from build123d import *

# Parameters (mm, degrees)
F0_W     = 41.1972631226
F0_H     = 41.1972631226
F1_DEPTH = 5
F0_R     = 1.65
F2_DEPTH = 2
F4_DEPTH = 4
F5_R     = 14.2181252649
F6_DEPTH = 1.001
F7_R     = 5


with BuildPart() as f1:
    # F0 (on Top) → F1 (new body)
    with BuildSketch(Plane.XY):
        Rectangle(F0_W, F0_H)
        Polygon((-16.9243157806, -12.35), (-13.5756842194, -12.35), (-11.9013684387, -15.25), (-13.5756842194, -18.15), (-16.9243157806, -18.15), (-18.5986315613, -15.25), align=None, mode=Mode.SUBTRACT)
        Polygon((13.5756842194, -12.35), (16.9243157806, -12.35), (18.5986315613, -15.25), (16.9243157806, -18.15), (13.5756842194, -18.15), (11.9013684387, -15.25), align=None, mode=Mode.SUBTRACT)
        Polygon((-18.5986315613, 15.25), (-16.9243157806, 18.15), (-13.5756842194, 18.15), (-11.9013684387, 15.25), (-13.5756842194, 12.35), (-16.9243157806, 12.35), align=None, mode=Mode.SUBTRACT)
        Polygon((13.5756842194, 18.15), (16.9243157806, 18.15), (18.5986315613, 15.25), (16.9243157806, 12.35), (13.5756842194, 12.35), (11.9013684387, 15.25), align=None, mode=Mode.SUBTRACT)
    extrude(amount=F1_DEPTH)

    # F0 (on Top) → F2 (join)
    with BuildSketch(Plane.XY):
        Polygon((-13.5756842194, 18.15), (-16.9243157806, 18.15), (-18.5986315613, 15.25), (-16.9243157806, 12.35), (-13.5756842194, 12.35), (-11.9013684387, 15.25), align=None)
        with Locations((-15.25, 15.25)):
            Circle(F0_R, mode=Mode.SUBTRACT)
        Polygon((18.5986315613, 15.25), (16.9243157806, 18.15), (13.5756842194, 18.15), (11.9013684387, 15.25), (13.5756842194, 12.35), (16.9243157806, 12.35), align=None)
        with Locations((15.25, 15.25)):
            Circle(F0_R, mode=Mode.SUBTRACT)
        Polygon((18.5986315613, -15.25), (16.9243157806, -12.35), (13.5756842194, -12.35), (11.9013684387, -15.25), (13.5756842194, -18.15), (16.9243157806, -18.15), align=None)
        with Locations((15.25, -15.25)):
            Circle(F0_R, mode=Mode.SUBTRACT)
        Polygon((-11.9013684387, -15.25), (-13.5756842194, -12.35), (-16.9243157806, -12.35), (-18.5986315613, -15.25), (-16.9243157806, -18.15), (-13.5756842194, -18.15), align=None)
        with Locations((-15.25, -15.25)):
            Circle(F0_R, mode=Mode.SUBTRACT)
    extrude(amount=F2_DEPTH)

    # F3 (on face) → F4 (cut)
    with BuildSketch(Plane(origin=(0, 0, 0), x_dir=(1, 0, 0), z_dir=(0, 0, -1))):
        with BuildLine():
            Line((-20.5986315613, 9.9013684387), (-20.5986315613, -9.9013684387))
            Line((-20.5986315613, -9.9013684387), (-15.25, -9.9013684387))
            ThreePointArc((-15.25, -9.9013684387), (-11.4679463529, -11.4679463529), (-9.9013684387, -15.25))
            Line((-9.9013684387, -15.25), (-9.9013684387, -20.5986315613))
            Line((-9.9013684387, -20.5986315613), (9.9013684387, -20.5986315613))
            Line((9.9013684387, -20.5986315613), (9.9013684387, -15.25))
            ThreePointArc((9.9013684387, -15.25), (11.4679463529, -11.4679463529), (15.25, -9.9013684387))
            Line((15.25, -9.9013684387), (20.5986315613, -9.9013684387))
            Line((20.5986315613, -9.9013684387), (20.5986315613, 9.9013684387))
            Line((20.5986315613, 9.9013684387), (15.25, 9.9013684387))
            ThreePointArc((15.25, 9.9013684387), (11.4679463529, 11.4679463529), (9.9013684387, 15.25))
            Line((9.9013684387, 15.25), (9.9013684387, 20.5986315613))
            Line((9.9013684387, 20.5986315613), (-9.9013684387, 20.5986315613))
            Line((-9.9013684387, 20.5986315613), (-9.9013684387, 15.25))
            ThreePointArc((-9.9013684387, 15.25), (-11.4679463529, 11.4679463529), (-15.25, 9.9013684387))
            Line((-15.25, 9.9013684387), (-20.5986315613, 9.9013684387))
        make_face()
    extrude(amount=-F4_DEPTH, mode=Mode.SUBTRACT)

    # F5 (on face) → F6 (cut, through all)
    with BuildSketch(Plane(origin=(0, 0, 4), x_dir=(1, 0, 0), z_dir=(0, 0, -1))):
        Circle(F5_R)
    extrude(amount=-F6_DEPTH, mode=Mode.SUBTRACT)

    # F7
    f7_edges = [f1.edges().sort_by_distance(p)[0] for p in [
        (-20.598632, 20.598632, 2.5),
        (20.598632, 20.598632, 2.5),
        (20.598632, -20.598632, 2.5),
        (-20.598632, -20.598632, 2.5),
        (-20.598632, -9.901368, 2),
        (-9.901368, -20.598632, 2),
        (-20.598632, 9.901368, 2),
        (-9.901368, 20.598632, 2),
        (9.901368, 20.598632, 2),
        (20.598632, 9.901368, 2),
        (20.598632, -9.901368, 2),
        (9.901368, -20.598632, 2),
    ]]
    fillet(f7_edges, radius=F7_R)


solid = f1.part
Read the model definition and answer for the solid it produces. Units are mm, in the model's axes. A direction names the side the tool comes from. Round coordinates to 2 decimals unless told otherwise and drop trailing zeros. Write each loop counter-clockwise with the first axis right and the second up, starting at its lowest first coordinate (ties: lowest second). Pieces come first, ordered by that corner, then holes. Notation, with made-up numbers: (30, 83.5) - (54, 83.5) arc R31 ccw to (54, 121.5) - close; hole circle Ø1 at (79, 3.5). An arc over 180 degrees is marked (long way). One line per question, with ' | ' between items. Start each with the question number.
1. Section C-C (z = 1.45) is taken. Give the number of separate pieces and of enclosed holes in the cut face, and give its area (3 significant figures).
2. Each of these flat-tipped pins is pushed along its axis until it touches: pin 1 (1 mm diameter, centred on y = 11, z = 1, fed in from -X); pin 2 (2 mm diameter, centred on x = -15.25, y = 15.25, fed in from -Z) (3 decimals); pin 3 (12.5 mm diameter, centred on x = 9.5, y = -1, fed in from -Z). Where does it stop, or does it pass through?
3. For faces 5 (the face through (12, -11, 2)), 6 (the face through (-5, 14, 5)), 7 (the face through (12.75, -16.72, 3.48)), 8 (the face through (-0.1, 20.599, 4.3)), 9 (the face through (11.4, -19.17, 2.03)), determine the directions among +Z, -Z, +X, -X, +Y, -Y from which every point of the face is accessible in a straight line to the end or side of a thin tool.
4. For a pull along Y with two mould halves and no side action, classify faces 1 (the face through (15, -12.35, 3)), 2 (the face through (-17, -16, 0)), 3 (the face through (-19.17, 19.1, 2.54)), 4 (the face through (-19.17, -11.4, 2.03)) as +Y half, -Y half, draft (parallel to the pull), parting line (faces both ways), or undercut.
5. Find the intervals of material crossed by probe 1 along Y at (x, z) = (15.5, 4.15); probe 2 along Y at (x, z) = (-15.25, 0.95); probe 3 along Y at (x, z) = (18, 3.1), in increasing order. Write a range as [from, to].
6. Section D-D (x = -11) is taken. Determine the outline of the cut face in (y, z).
7. Section A-A (y = 0) is taken. Determine the outline of the cut face in (x, z), and give its area (3 significant figures).
Filled in:
1) separate pieces: 4 | enclosed holes: 4 | area: 335 mm²
2) pin 1: x = -19.26 | pin 2: through | pin 3: z = 4
3) face 5: -Z | face 6: +Z, +X, -X, +Y, -Y | face 7: +Z | face 8: +Z, -Z, +X, -X, +Y | face 9: -Z, -Y
4) face 1: undercut | face 2: draft | face 3: +Y half | face 4: undercut
5) probe 1: [-20.6, -18.15], [-12.35, 12.35], [18.15, 20.6] | probe 2: [-20.6, -16.9], [-13.6, -9.9], [9.9, 13.6], [16.9, 20.6] | probe 3: [-19.98, -16.29], [-14.21, -10.52], [10.52, 14.21], [16.29, 19.98]
6) outline: (-20.6, 4) - (-18.73, 4) - (-18.73, 0) - (-12, 0) - (-12, 4) - (-9.01, 4) - (-9.01, 5) - (-20.6, 5) - close; (9.01, 4) - (12, 4) - (12, 0) - (18.73, 0) - (18.73, 4) - (20.6, 4) - (20.6, 5) - (9.01, 5) - close
7) outline: (-20.6, 4) - (-14.22, 4) - (-14.22, 5) - (-20.6, 5) - close; (14.22, 4) - (20.6, 4) - (20.6, 5) - (14.22, 5) - close | area: 12.8 mm²
